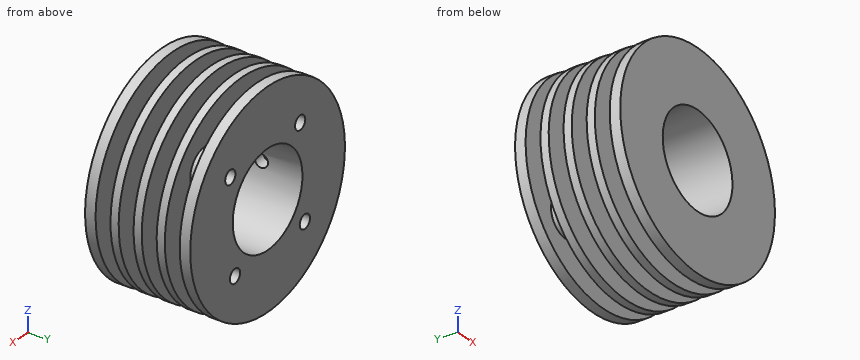
```python
from build123d import *

# Parameters (mm, degrees)
SKETCH1_R                        = 31.75
SKETCH1_R_2                      = 14.3129
BOSS_EXTRUDE1_DEPTH              = 31.75
SKETCH2_W                        = 13.97
SKETCH2_H                        = 4.5
BOSS_EXTRUDE2_START              = -7.675
BOSS_EXTRUDE2_DEPTH              = 4.5
CUT_EXTRUDE2_REACH               = 56.993
CUT_EXTRUDE2_END_RADIUS          = 17.78
SKETCH8_R                        = 2
CUT_EXTRUDE3_REACH               = 56.993
CUT_EXTRUDE3_END_RADIUS          = 17.78
SKETCH9_R                        = 2
SKETCH10_R                       = 1
CUT_EXTRUDE4_DEPTH               = 10.141666667
TAP_DRILL_FOR_M5X0_8_TAP1_REACH  = 74.51
TAP_DRILL_FOR_M5X0_8_TAP1_BORE_R = 2.1


# Read off the part's stored shape, not the designer's step: Boss-Extrude2
with BuildPart() as part:
    # Sketch1 → Boss-Extrude1 (new body)
    with BuildSketch(Plane(origin=(0, 0, 0), x_dir=(1, 0, 0), z_dir=(0, 1, 0))):
        with Locations(Location((0, 0, 0), (0, 0, 270))):
            Circle(SKETCH1_R)
        with Locations(Location((0, 0, 0), (0, 0, 270))):
            Circle(SKETCH1_R_2, mode=Mode.SUBTRACT)
    extrude(amount=BOSS_EXTRUDE1_DEPTH)

    # Sketch2 → Cut-Revolve2 (revolve, cut)
    with BuildSketch(Plane.XY, mode=Mode.PRIVATE) as cut_revolve2_sk:
        with Locations((24.765, 26.325)):
            Rectangle(SKETCH2_W, SKETCH2_H)
        with Locations((24.765, 12.391666667)):
            Rectangle(SKETCH2_W, SKETCH2_H)
        with Locations((24.765, 5.425)):
            Rectangle(SKETCH2_W, SKETCH2_H)
        with Locations((24.765, 19.358333333)):
            Rectangle(SKETCH2_W, SKETCH2_H)
    revolve(cut_revolve2_sk.sketch.rotate(Axis((0, 0, 0), (0, 1, 0)), 90), axis=Axis((0, 0, 0), (0, 1, 0)), mode=Mode.SUBTRACT)

    # Boss-Extrude2 outline → Boss-Extrude2 (add)
    with BuildSketch(Plane(origin=(0, 31.75, 0), x_dir=(1, 0, 0), z_dir=(0, 1, 0)).offset(BOSS_EXTRUDE2_START)):
        with BuildLine():
            ThreePointArc((-10.269067687, -20.446529483), (-6.799835435, -18.70202978), (-3.105226449, -17.506740665))
            ThreePointArc((-3.105226449, -17.506740665), (-11.698828781, -13.38901808), (-16.932025536, -5.425395031))
            ThreePointArc((-16.932025536, -5.425395031), (-17.620944734, -9.246944713), (-18.884341927, -12.918821503))
            ThreePointArc((-18.884341927, -12.918821503), (-17.322622903, -19.825310342), (-10.269067687, -20.446529483))
        make_face()
        with BuildLine():
            ThreePointArc((17.506740665, -3.105226449), (13.38901808, -11.698828781), (5.425395031, -16.932025536))
            ThreePointArc((5.425395031, -16.932025536), (9.246944713, -17.620944734), (12.918821503, -18.884341927))
            ThreePointArc((12.918821503, -18.884341927), (19.825310342, -17.322622903), (20.446529483, -10.269067687))
            ThreePointArc((20.446529483, -10.269067687), (18.70202978, -6.799835435), (17.506740665, -3.105226449))
        make_face()
        with BuildLine():
            ThreePointArc((-20.446529483, 10.269067687), (-18.70202978, 6.799835435), (-17.506740665, 3.105226449))
            ThreePointArc((-17.506740665, 3.105226449), (-13.38901808, 11.698828781), (-5.425395031, 16.932025536))
            ThreePointArc((-5.425395031, 16.932025536), (-9.246944713, 17.620944734), (-12.918821503, 18.884341927))
            ThreePointArc((-12.918821503, 18.884341927), (-19.825310342, 17.322622903), (-20.446529483, 10.269067687))
        make_face()
        with BuildLine():
            ThreePointArc((10.269067687, 20.446529483), (6.799835435, 18.70202978), (3.105226449, 17.506740665))
            ThreePointArc((3.105226449, 17.506740665), (11.698828781, 13.38901808), (16.932025536, 5.425395031))
            ThreePointArc((16.932025536, 5.425395031), (17.620944734, 9.246944713), (18.884341927, 12.918821503))
            ThreePointArc((18.884341927, 12.918821503), (17.322622903, 19.825310342), (10.269067687, 20.446529483))
        make_face()
    extrude(amount=BOSS_EXTRUDE2_DEPTH)

    # Cut-Extrude2: up to this cylinder (the profile starts inside it)
    cut_extrude2_end = Plane(origin=(0, 19.358333, 0), z_dir=(0, -1, 0)) * Cylinder(CUT_EXTRUDE2_END_RADIUS, 150.546, mode=Mode.PRIVATE)
    # Sketch8 → Cut-Extrude2 (cut, up to the surface)
    with BuildSketch(Plane.XY, mode=Mode.PRIVATE) as cut_extrude2_sk1:
        with Locations(Location((0, 19.358333333, 0), (0, 0, 180))):
            Circle(SKETCH8_R)
    cut_extrude2_tool1 = extrude(cut_extrude2_sk1.sketch, amount=CUT_EXTRUDE2_REACH, mode=Mode.PRIVATE) & cut_extrude2_end
    add(cut_extrude2_tool1.solids().sort_by_distance((0, 19.358333, 0))[0], mode=Mode.SUBTRACT)

    # Cut-Extrude3: up to this cylinder (the profile starts inside it)
    cut_extrude3_end = Plane(origin=(0, 19.358333, 0), z_dir=(0, -1, 0)) * Cylinder(CUT_EXTRUDE3_END_RADIUS, 150.546, mode=Mode.PRIVATE)
    # Sketch9 → Cut-Extrude3 (cut, up to the surface)
    with BuildSketch(Plane(origin=(0, 0, 0), x_dir=(0, 0, -1), z_dir=(1, 0, 0)), mode=Mode.PRIVATE) as cut_extrude3_sk1:
        with Locations((0, 19.358333333)):
            Circle(SKETCH9_R)
    cut_extrude3_tool1 = extrude(cut_extrude3_sk1.sketch, amount=-CUT_EXTRUDE3_REACH, mode=Mode.PRIVATE) & cut_extrude3_end
    add(cut_extrude3_tool1.solids().sort_by_distance((0, 19.358333, 0))[0], mode=Mode.SUBTRACT)

    # Sketch10 → Cut-Extrude4 (cut)
    with BuildSketch(Plane(origin=(0, 31.75, 0), x_dir=(1, 0, 0), z_dir=(0, 1, 0))):
        with Locations(Location((15.301734948, -13.370090036, 0), (0, 0, 270))):
            Circle(SKETCH10_R)
        with Locations(Location((13.370090036, 15.301734948, 0), (0, 0, 270))):
            Circle(SKETCH10_R)
        with Locations(Location((-15.301734948, 13.370090036, 0), (0, 0, 270))):
            Circle(SKETCH10_R)
        with Locations(Location((-13.370090036, -15.301734948, 0), (0, 0, 270))):
            Circle(SKETCH10_R)
    extrude(amount=-CUT_EXTRUDE4_DEPTH, mode=Mode.SUBTRACT)

    # Tap Drill for M5x0.8 Tap1 bore (on position points) → Tap Drill for M5x0.8 Tap1 (cut, up to next)
    with BuildSketch(Plane(origin=(15.301734948, 31.75, 13.370090036), x_dir=(0, 0, 1), z_dir=(0, 1, 0)), mode=Mode.PRIVATE) as tap_drill_for_m5x0_8_tap1_sk1:
        Circle(TAP_DRILL_FOR_M5X0_8_TAP1_BORE_R)
    tap_drill_for_m5x0_8_tap1_tool1 = extrude(tap_drill_for_m5x0_8_tap1_sk1.sketch, amount=-TAP_DRILL_FOR_M5X0_8_TAP1_REACH, mode=Mode.PRIVATE) & part.part
    # Tap Drill for M5x0.8 Tap1 bore (on position points) → Tap Drill for M5x0.8 Tap1 (cut, up to next)
    with BuildSketch(Plane(origin=(15.301734948, 31.75, 13.370090036), x_dir=(0, 0, 1), z_dir=(0, 1, 0)), mode=Mode.PRIVATE) as tap_drill_for_m5x0_8_tap1_sk2:
        with Locations((1.931644912, -28.671824984)):
            Circle(TAP_DRILL_FOR_M5X0_8_TAP1_BORE_R)
    tap_drill_for_m5x0_8_tap1_tool2 = extrude(tap_drill_for_m5x0_8_tap1_sk2.sketch, amount=-TAP_DRILL_FOR_M5X0_8_TAP1_REACH, mode=Mode.PRIVATE) & part.part
    # Tap Drill for M5x0.8 Tap1 bore (on position points) → Tap Drill for M5x0.8 Tap1 (cut, up to next)
    with BuildSketch(Plane(origin=(15.301734948, 31.75, 13.370090036), x_dir=(0, 0, 1), z_dir=(0, 1, 0)), mode=Mode.PRIVATE) as tap_drill_for_m5x0_8_tap1_sk3:
        with Locations((-26.740180072, -30.603469896)):
            Circle(TAP_DRILL_FOR_M5X0_8_TAP1_BORE_R)
    tap_drill_for_m5x0_8_tap1_tool3 = extrude(tap_drill_for_m5x0_8_tap1_sk3.sketch, amount=-TAP_DRILL_FOR_M5X0_8_TAP1_REACH, mode=Mode.PRIVATE) & part.part
    # Tap Drill for M5x0.8 Tap1 bore (on position points) → Tap Drill for M5x0.8 Tap1 (cut, up to next)
    with BuildSketch(Plane(origin=(15.301734948, 31.75, 13.370090036), x_dir=(0, 0, 1), z_dir=(0, 1, 0)), mode=Mode.PRIVATE) as tap_drill_for_m5x0_8_tap1_sk4:
        with Locations((-28.671824984, -1.931644912)):
            Circle(TAP_DRILL_FOR_M5X0_8_TAP1_BORE_R)
    tap_drill_for_m5x0_8_tap1_tool4 = extrude(tap_drill_for_m5x0_8_tap1_sk4.sketch, amount=-TAP_DRILL_FOR_M5X0_8_TAP1_REACH, mode=Mode.PRIVATE) & part.part
    add(tap_drill_for_m5x0_8_tap1_tool1.solids().sort_by_distance((15.301735, 31.75, 13.37009))[0], mode=Mode.SUBTRACT)
    add(tap_drill_for_m5x0_8_tap1_tool2.solids().sort_by_distance((-13.37009, 31.75, 15.301735))[0], mode=Mode.SUBTRACT)
    add(tap_drill_for_m5x0_8_tap1_tool3.solids().sort_by_distance((-15.301735, 31.75, -13.37009))[0], mode=Mode.SUBTRACT)
    add(tap_drill_for_m5x0_8_tap1_tool4.solids().sort_by_distance((13.37009, 31.75, -15.301735))[0], mode=Mode.SUBTRACT)


solid = part.part
```
For this review, take the finished solid that the model builds, in its own axes (mm). Coordinates: 2 decimals unless noted, no trailing zeros. Loops run counter-clockwise (first coordinate to the right, second up) from the corner with the lowest first, then second, coordinate; pieces in that order, holes last.
1. Add section A-A, the plane y = 20.5. Give the boundary of the cut face in (x, z), then the cut area to 3 significant figures.
2. Add section C-C, the plane y = 12.5. Give the boundary of the cut face in (x, z).
3. For line 1 (Y direction, x = -29, z = -3.5) (3 decimals); line 2 (X direction, y = 14, z = 0); line 3 (X direction, y = 5, z = 5), list the stretches that pass through material, from the lowest coordinate up.
4. Add section B-B, the plane x = 0. Count the separate pieces of the cut face and the enclosed holes in it, then the cut area to 3 significant figures.
5. Insertion check: P1, Ø4, axis at y = 21.5, z = -5.5, coming from the +X side; P2, Ø4, axis at y = 25.5, z = -20, coming from the +X side; P3, Ø10, axis at x = -11.5, y = 20.5, coming from the -Z side. Each pin has a flat end and moves straight along its axis. Give the tip position at first contact, or say it passes through.
Result:
1. outline: (-17.7, -1.64) arc R17.78 ccw (long way) to (1.64, 17.7) - (1.64, 14.22) arc R14.31 cw (long way) to (-14.22, -1.64) - close; (-17.7, 1.64) - (-14.22, 1.64) arc R14.31 cw to (-1.64, 14.22) - (-1.64, 17.7) arc R17.78 ccw to start
1. area: 327 mm2
2. outline: circle Ø35.56 at (0, 0); hole circle Ø28.63 at (0, 0)
3. line 1: y = 0 to 3.175, 7.675 to 10.142, 14.642 to 17.108, 21.608 to 24.075, 28.575 to 31.75
3. line 2: x = -17.78 to -14.31, 14.31 to 17.78
3. line 3: x = -17.06 to -13.41, 13.41 to 17.06
4. separate pieces: 3
4. enclosed holes: 0
4. area: 590 mm2
5. P1: stops at x = 31.56
5. P2: stops at x = 25.73
5. P3: stops at z = -31.05
